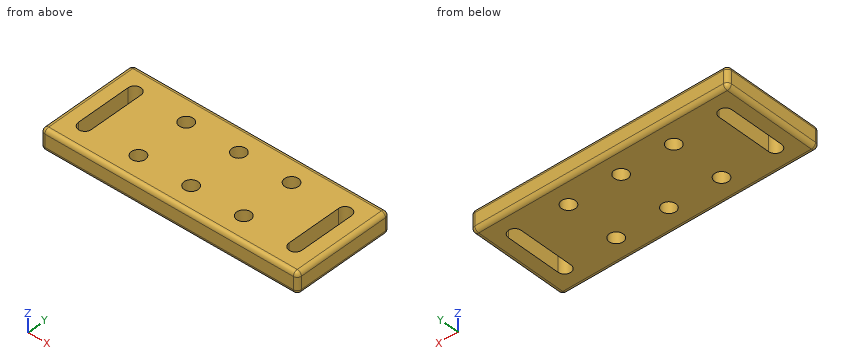
```python
from build123d import *

# Parameters (mm, degrees)
SKETCH_W    = 122
SKETCH_H    = 48
PAD_DEPTH   = 10
SKETCH001_R = 3.3
HOLE_DEPTH  = 10.001
FILLET_R    = 2
FILLET001_R = 2
FILLET002_R = 2
FILLET003_R = 2
FILLET004_R = 2


with BuildPart() as part:
    # Sketch → Pad (new body)
    with BuildSketch(Plane.XY):
        Rectangle(SKETCH_W, SKETCH_H)
        with BuildLine():
            ThreePointArc((53.05, 13), (50, 16.05), (46.95, 13))
            Line((46.95, 13), (46.95, -13))
            ThreePointArc((46.95, -13), (50, -16.05), (53.05, -13))
            Line((53.05, -13), (53.05, 13))
        make_face(mode=Mode.SUBTRACT)
        with BuildLine():
            ThreePointArc((-46.95, 13), (-50, 16.05), (-53.05, 13))
            Line((-53.05, 13), (-53.05, -13))
            ThreePointArc((-53.05, -13), (-50, -16.05), (-46.95, -13))
            Line((-46.95, -13), (-46.95, 13))
        make_face(mode=Mode.SUBTRACT)
    extrude(amount=PAD_DEPTH)

    # Sketch001 (on Face14 of Pad) → Hole (cut, through all)
    with BuildSketch(Plane.XY.offset(10)):
        with Locations((0, 12.5)):
            Circle(SKETCH001_R)
        with Locations((25, 12.5)):
            Circle(SKETCH001_R)
        with Locations((0, -12.5)):
            Circle(SKETCH001_R)
        with Locations((25, -12.5)):
            Circle(SKETCH001_R)
        with Locations((-25, 12.5)):
            Circle(SKETCH001_R)
        with Locations((-25, -12.5)):
            Circle(SKETCH001_R)
    extrude(amount=-HOLE_DEPTH, mode=Mode.SUBTRACT)

    # Fillet
    fillet_edges = [part.edges().sort_by_distance(p)[0] for p in [
        (0, 24, 10),
    ]]
    fillet(fillet_edges, radius=FILLET_R)

    # Fillet001
    fillet001_edges = [part.edges().sort_by_distance(p)[0] for p in [
        (0, -24, 10),
    ]]
    fillet(fillet001_edges, radius=FILLET001_R)

    # Fillet002
    fillet002_edges = [part.edges().sort_by_distance(p)[0] for p in [
        (-61, 0, 10),
    ]]
    fillet(fillet002_edges, radius=FILLET002_R)

    # Fillet003
    fillet003_edges = [part.edges().sort_by_distance(p)[0] for p in [
        (61, 0, 10),
    ]]
    fillet(fillet003_edges, radius=FILLET003_R)

    # Fillet004
    fillet004_edges = [part.edges().sort_by_distance(p)[0] for p in [
        (0, -24, 0),
    ]]
    fillet(fillet004_edges, radius=FILLET004_R)


solid = part.part
```
Build history of the part. All positions in model axes, mm. Round coordinates to 2 decimals unless told otherwise and drop trailing zeros. Loops run counter-clockwise (first coordinate to the right, second up) from the corner with the lowest first, then second, coordinate; pieces in that order, holes last.
Item 1: Saw through at C-C (z = 6). State how many separate pieces and enclosed holes the cut face has, then the cut area to 3 significant figures.
Item 2: Saw through at B-B (x = 0). List the corners of the cut face in (y, z), then the cut area to 3 significant figures.
Item 3: Saw through at D-D (x = -50). List the corners of the cut face in (y, z), then the cut area to 3 significant figures.
Item 4: Drill centre lines: line 1 along X through (y, z) = (-2, 5.25); line 2 along Y through (x, z) = (25, 5.75); line 3 along X through (y, z) = (4, 8.75). Where is each one in solid material? Low to high.
Item 5: Saw through at A-A (y = -5.5). List the corners of the cut face in (x, z), then the cut area to 3 significant figures.
Worked answers:
1. separate pieces: 1
1. enclosed holes: 8
1. area: 5,270 mm2
2. outline: (-24, 2) arc R2 ccw to (-22, 0) - (-15.8, 0) - (-15.8, 10) - (-22, 10) arc R2 ccw to (-24, 8) - close; (-9.2, 0) - (9.2, 0) - (9.2, 10) - (-9.2, 10) - close; (15.8, 0) - (22, 0) arc R2 ccw to (24, 2) - (24, 8) arc R2 ccw to (22, 10) - (15.8, 10) - close
2. area: 345 mm2
3. outline: (-24, 2) arc R2 ccw to (-22, 0) - (-16.05, 0) - (-16.05, 10) - (-22, 10) arc R2 ccw to (-24, 8) - close; (16.05, 0) - (22, 0) arc R2 ccw to (24, 2) - (24, 8) arc R2 ccw to (22, 10) - (16.05, 10) - close
3. area: 156 mm2
4. line 1: x = -61 to -53.05, -46.95 to 46.95, 53.05 to 61
4. line 2: y = -24 to -15.8, -9.2 to 9.2, 15.8 to 24
4. line 3: x = -60.85 to -53.05, -46.95 to 46.95, 53.05 to 60.85
5. outline: (-61, 2) arc R2 ccw to (-59, 0) - (-53.05, 0) - (-53.05, 10) - (-59, 10) arc R2 ccw to (-61, 8) - close; (-46.95, 0) - (46.95, 0) - (46.95, 10) - (-46.95, 10) - close; (53.05, 0) - (59, 0) arc R2 ccw to (61, 2) - (61, 8) arc R2 ccw to (59, 10) - (53.05, 10) - close
5. area: 1,090 mm2
